Autodesk Inventor part; units mm, degrees
ref_plane "YZ Plane" through (0, 0, 0) normal (1, 0, 0) x (0, 1, 0)
ref_plane "XZ Plane" through (0, 0, 0) normal (0, 1, 0) x (-1, 0, 0)
ref_plane "XY Plane" through (0, 0, 0) normal (0, 0, 1) x (1, 0, 0)
sketch "Эскиз1" plane through (0, 0, 0) normal (0, 1, 0) x (-1, 0, 0)
  arc A0 (29.8038, -3) -> (29.8038, 3) centre (35, 0) ccw
  line L0 (30.0057, 0) -> (28.0258, 0)
  circle A1 centre (35, 0) radius 1.9
  arc A2 (-29.8038, 3) -> (-29.8038, -3) centre (-35, 0) ccw
  line L1 (-29.8038, -3) -> (29.8038, -3)
  line L2 (-29.8038, 3) -> (29.8038, 3)
  circle A3 centre (-35, 0) radius 1.9
  line L3 (32.9518, 0) -> (37.6343, 0) construction
  line L4 (14.11, -3) -> (14.11, 3)
  line L5 (0, -3) -> (0, 3)
  point P0 (0, 0)
  point P1 (25.2378, -3)
  point P2 (25.2378, 3)
  point P3 (0, 0)
  dimension "d2" = 6
  dimension "d3" = 35
  dimension "d4" = 3.8
  dimension "d9" = 6
extrude "Выдавливание1" add sketch "Эскиз1" along normal mid plane 3
fillet "Сопряжение1" radius 10 4 edges at (-29.8038, 0, 3) (-29.8038, 0, -3) (29.8038, 0, -3) (29.8038, 0, 3)
properties part number "Рычаг"
CAD build for the part. Positions are in the model's coordinates, mm. A direction names the side the tool comes from. Round coordinates to 2 decimals unless told otherwise and drop trailing zeros. Loops run counter-clockwise (first coordinate to the right, second up) from the corner with the lowest first, then second, coordinate; pieces in that order, holes last. Notation, with made-up numbers: (-33, 62.25) - (-12, 62.25) arc R17 cw to (-12, 90.25) - close; hole circle Ø2 at (-1, -13). An arc over 180 degrees is marked (long way). Return JSON: item names as keys, results as strings. Group by question number.
Q1. Two-plate mould, pull along X, no slides. Class faces 1 (the face through (1, -1.5, 0)), 2 (the face through (-28.693, 0.021, 3.467)): +X half, -X half, draft (parallel to the pull), parting line (faces both ways), or undercut.
Q2. Band-saw the part on D-D on x = 19. Give the cut face in (y, z).
Q3. Flat gauge pins, fed straight in: pin 1 Ø1.5 at (x, y) = (11, 0.5) entering from -Z; pin 2 Ø1.5 at (y, z) = (0, -1) entering from +X; pin 3 Ø3.5 at (x, z) = (-35, 0) entering from -Y. Where does each tip first touch, or does it go through?
Q4. Band-saw the part on C-C on y = 0.3. Give the cut face in (x, z).
Q5. Drill centre lines: line 1 along Z through (x, y) = (35, -0.65); line 2 along X through (y, z) = (0.95, 4); line 3 along Z through (x, y) = (34, 0.6). Where is each one in solid material? Low to high. Write a range as [from, to].
Q6. Band-saw the part on A-A on z = 0. Give the cut face in (x, y).
Q7. Band-saw the part on B-B on x = 35. Give the cut face in (y, z), plus the area to 3 significant figures.
Q8. Tool access for faces 3 (the face through (41, 0, 0)), 4 (the face through (0, 0, 3)), 5 (the face through (-28.8, 0, -3.5)): list every direction of +Z, -Z, +X, -X, +Y, -Y with a clear straight run to the whole face (end or side of a thin tool).
Solutions:
{
 "1": {"face 1": "draft", "face 2": "undercut"},
 "2": {"outline": "(-1.5, -3) - (1.5, -3) - (1.5, 3) - (-1.5, 3) - close"},
 "3": {"pin 1": "stops at z = -3", "pin 2": "stops at x = 40.99", "pin 3": "passes through"},
 "4": {"outline": "(-31.5, -4.88) arc R10 cw to (-25.67, -3) - (25.67, -3) arc R10 cw to (31.5, -4.88) arc R6 ccw (long way) to (31.5, 4.88) arc R10 cw to (25.67, 3) - (-25.67, 3) arc R10 cw to (-31.5, 4.88) arc R6 ccw (long way) to start; hole circle Ø3.8 at (-35, 0); hole circle Ø3.8 at (35, 0)"},
 "5": {"line 1": "z = [-6, -1.9], [1.9, 6]", "line 2": "x = [-39.47, -30.03], [30.03, 39.47]", "line 3": "z = [-5.92, -1.62], [1.62, 5.92]"},
 "6": {"outline": "(-41, -1.5) - (-36.9, -1.5) - (-36.9, 1.5) - (-41, 1.5) - close; (-33.1, -1.5) - (33.1, -1.5) - (33.1, 1.5) - (-33.1, 1.5) - close; (36.9, -1.5) - (41, -1.5) - (41, 1.5) - (36.9, 1.5) - close"},
 "7": {"outline": "(-1.5, -6) - (1.5, -6) - (1.5, -1.9) - (-1.5, -1.9) - close; (-1.5, 1.9) - (1.5, 1.9) - (1.5, 6) - (-1.5, 6) - close", "area": "24.6 mm^2"},
 "8": {"face 3": "+Y, -Y", "face 4": "+Z, +Y, -Y", "face 5": "-Z, +Y, -Y"}
}
